For this review, take the finished solid that the model builds, in its own axes (mm). A direction names the side the tool comes from. Coordinates: 2 decimals unless noted, no trailing zeros. Write each loop counter-clockwise with the first axis right and the second up, starting at its lowest first coordinate (ties: lowest second). Pieces come first, ordered by that corner, then holes. Notation, with made-up numbers: M 4.25,12.25 L 15.25,12.25 A37 cw 15.25,51.25 Z; hole C -14.75,27 d1. An arc over 180 degrees is marked long. Return JSON: item names as keys, results as strings.
```python
from build123d import *

# Parameters (mm, degrees)
SKETCH1_W                = 37
SKETCH1_H                = 37
BOSS_EXTRUDE1_DEPTH      = 100
BOSS_EXTRUDE2_DEPTH      = 6
BOSS_EXTRUDE2_DEPTH_BACK = 43
BOSS_EXTRUDE3_DEPTH      = 6
BOSS_EXTRUDE3_DEPTH_BACK = 43


with BuildPart() as part:
    # Sketch1 → Boss-Extrude1 (new body)
    with BuildSketch(Plane(origin=(0, 0, 0), x_dir=(1, 0, 0), z_dir=(0, 1, 0))):
        Rectangle(SKETCH1_W, SKETCH1_H)
    extrude(amount=BOSS_EXTRUDE1_DEPTH)

    # Sketch2 → Boss-Extrude2 (add, two sides: drawn at the far end of the back side and taken through both)
    with BuildSketch(Plane.ZY.offset(18.5).offset(-BOSS_EXTRUDE2_DEPTH_BACK)):
        Polygon((2.947677665, 14.601477232), (5.53699788, 19.086311402), (2.947677665, 23.571145571), (-2.230962765, 23.571145571), (-4.82028298, 19.086311402), (-2.230962765, 14.601477232), align=None)
        Polygon((2.265923415, 31.999576723), (4.85524363, 36.484410892), (2.265923415, 40.969245062), (-2.912717015, 40.969245062), (-5.50203723, 36.484410892), (-2.912717015, 31.999576723), align=None)
        Polygon((2.148184021, 50.736854031), (4.737504236, 55.221688201), (2.148184021, 59.70652237), (-3.030456409, 59.70652237), (-5.619776624, 55.221688201), (-3.030456409, 50.736854031), align=None)
        Polygon((2.302648162, 69.385244476), (4.891968377, 73.870078646), (2.302648162, 78.354912815), (-2.875992268, 78.354912815), (-5.465312483, 73.870078646), (-2.875992268, 69.385244476), align=None)
    extrude(amount=BOSS_EXTRUDE2_DEPTH + BOSS_EXTRUDE2_DEPTH_BACK)

    # Sketch3 → Boss-Extrude3 (add, two sides: drawn at the far end of the back side and taken through both)
    with BuildSketch(Plane.XY.offset(18.5).offset(-BOSS_EXTRUDE3_DEPTH_BACK)):
        Polygon((2.683056757, 13.510428104), (5.640179705, 18.315850916), (2.957122948, 23.279505916), (-2.683056757, 23.437738105), (-5.640179705, 18.632315293), (-2.957122948, 13.668660293), align=None)
        Polygon((2.957122948, 30.681991349), (5.824876018, 35.910513005), (2.730719975, 41.008320843), (-3.231189138, 40.877607026), (-6.098942208, 35.64908537), (-3.004786166, 30.551277532), align=None)
        Polygon((2.730719975, 50.402458514), (5.595494766, 55.367833024), (2.727741696, 60.331488025), (-3.004786166, 60.329768515), (-5.869560957, 55.364394004), (-3.001807886, 50.400739003), align=None)
        Polygon((2.727741696, 68.244785948), (5.709440822, 73.275947245), (2.843176891, 78.373755084), (-3.004786166, 78.440401625), (-5.986485292, 73.409240328), (-3.120221361, 68.311432489), align=None)
    extrude(amount=BOSS_EXTRUDE3_DEPTH + BOSS_EXTRUDE3_DEPTH_BACK)


solid = part.part
```
1. We need section B-B (z = -21.5). State the section outline as (x, y) points.
Checks:
{"outline": "M -6.1,35.65 L -3,30.55 L 2.96,30.68 L 5.82,35.91 L 2.73,41.01 L -3.23,40.88 Z; M -5.99,73.41 L -3.12,68.31 L 2.73,68.24 L 5.71,73.28 L 2.84,78.37 L -3,78.44 Z; M -5.87,55.36 L -3,50.4 L 2.73,50.4 L 5.6,55.37 L 2.73,60.33 L -3,60.33 Z; M -5.64,18.63 L -2.96,13.67 L 2.68,13.51 L 5.64,18.32 L 2.96,23.28 L -2.68,23.44 Z"}
2. We need section A-A (x = 19.5). State the section outline as (y, z) points.
Checks:
{"outline": "M 14.6,-2.23 L 19.09,-4.82 L 23.57,-2.23 L 23.57,2.95 L 19.09,5.54 L 14.6,2.95 Z; M 32,-2.91 L 36.48,-5.5 L 40.97,-2.91 L 40.97,2.27 L 36.48,4.86 L 32,2.27 Z; M 50.74,-3.03 L 55.22,-5.62 L 59.71,-3.03 L 59.71,2.15 L 55.22,4.74 L 50.74,2.15 Z; M 69.39,-2.88 L 73.87,-5.47 L 78.35,-2.88 L 78.35,2.3 L 73.87,4.89 L 69.39,2.3 Z"}
3. Draft analysis for pull direction Y (two halves, no side actions). For faces 4 (the face through (-4.573, 70.896, 21.458)), 5 (the face through (-24.5, 19, 0)), 6 (the face through (0, 0, 0)), state which applies: +Y half, -Y half, draft (parallel to the pull), parting line (faces both ways), or undercut.
Checks:
{"face 4": "undercut", "face 5": "draft", "face 6": "-Y half"}
4. We need section C-C (y = 71). State the section outline as (x, z) points, plus the area to 3 significant figures.
Checks:
{"outline": "M -24.5,-3.81 L -18.5,-3.81 L -18.5,-18.5 L -4.63,-18.5 L -4.63,-24.5 L 4.36,-24.5 L 4.36,-18.5 L 18.5,-18.5 L 18.5,-3.81 L 24.5,-3.81 L 24.5,3.23 L 18.5,3.23 L 18.5,18.5 L 4.36,18.5 L 4.36,24.5 L -4.63,24.5 L -4.63,18.5 L -18.5,18.5 L -18.5,3.23 L -24.5,3.23 Z", "area": "1,560 mm2"}
5. Clearance check with flat-ended pins moving along their axes: pin 1 Ø2.5 at (x, z) = (-22.5, 1) entering from -Y; pin 2 Ø3 at (y, z) = (25.5, 9.5) entering from +X; pin 3 Ø1.6 at (x, z) = (21.5, -1.5) entering from +Y. State where each tip first meets the part, or that it passes through.
Checks:
{"pin 1": "y = 14.6", "pin 2": "x = 18.5", "pin 3": "y = 78.35"}
6. We need section D-D (x = -15.5). State the section outline as (y, z) points.
Checks:
{"outline": "M 0,-18.5 L 100,-18.5 L 100,18.5 L 0,18.5 Z"}
7. Wall thickness on L1, parallel to Y at x = 2.5, z = -19.5; L2, parallel to Y at x = -3.5, z = -21; L3, parallel to X at y = 57, z = 15: over which ranges is each line inside the solid? List them lowest first. Write a range as from..to.
Checks:
{"L1": "13.52..23.29, 30.67..41, 50.4..60.33, 68.25..78.38", "L2": "14.67..22.11, 31.37..40.39, 51.26..59.47, 68.99..77.6", "L3": "-18.5..18.5"}
8. For faces 1 (the face through (21.542, 52.948, 3.425)), 2 (the face through (21.542, 76.144, -4.153)), 3 (the face through (-21.458, 57.495, -4.307)), list the 3-axis set-ups (+Z, -Z, +X, -X, +Y, -Y) from which the entire face can be reached by the end or side of a thin tool; tool diameter is ignored.
Checks:
{"face 1": "+Z, +X", "face 2": "-Z, +X, +Y", "face 3": "-Z, -X"}
